Design review of the part built by this model. Coordinates are the model's own, in mm. Face numbers are marked on the shaded views. Round coordinates to 2 decimals unless told otherwise and drop trailing zeros. Order: outer loops, then holes, each group sorted by start corner. A loop starts at its lowest first (then second) coordinate and runs counter-clockwise, first axis right, second up. Notation, with made-up numbers: (-38, -9.5) - (-21, -9.5) arc R37 ccw to (-21, 29.5) - close; hole circle Ø1 at (-22.5, 45). An arc over 180 degrees is marked (long way). Write item = value, one per line.
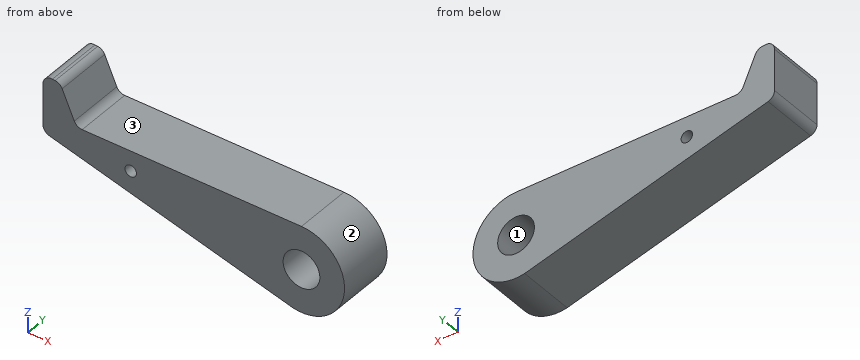
from build123d import *

# Parameters (mm, degrees)
SKETCH1_R           = 3.2
SKETCH1_R_2         = 1
BOSS_EXTRUDE1_DEPTH = 10
FILLET1_R           = 1.5


with BuildPart() as part:
    # Sketch1 → Boss-Extrude1 (new body)
    with BuildSketch(Plane(origin=(0, 0, 0), x_dir=(1, 0, 0), z_dir=(0, 1, 0))):
        with BuildLine():
            Line((0, 45), (43.494782903, 56.541397673))
            ThreePointArc((43.494782903, 56.541397673), (52.461753069, 49.950461527), (45, 41.69399531))
            Line((45, 41.69399531), (5.847258058, 41.69399531))
            Line((5.847258058, 41.69399531), (2.984330404, 35.306222204))
            Line((2.984330404, 35.306222204), (0, 35))
            Line((0, 35), (0, 45))
        make_face()
        with Locations(Location((45, 49.19399531, 0), (0, 0, 270))):
            Circle(SKETCH1_R, mode=Mode.SUBTRACT)
        with Locations(Location((15.270504009, 45.174409747, 0), (0, 0, 270))):
            Circle(SKETCH1_R_2, mode=Mode.SUBTRACT)
    extrude(amount=BOSS_EXTRUDE1_DEPTH)

    # Fillet1
    fillet1_edges = [part.edges().sort_by_distance(p)[0] for p in [
        (5.847258058, 5, -41.69399531),
        (2.984330404, 5, -35.306222204),
        (0, 5, -35),
        (0, 5, -45),
    ]]
    fillet(fillet1_edges, radius=FILLET1_R)


solid = part.part
Item 1: Take a section at A-A, the plane y = 1.25. State the section outline as (x, z) points, and give its area (3 significant figures).
Data:
outline = (0, -43.85) arc R1.5 ccw to (1.12, -45.3) - (43.49, -56.54) arc R7.5 ccw (long way) to (45, -41.69) - (6.82, -41.69) arc R1.5 cw to (5.45, -40.81) - (3.34, -36.1) arc R1.5 ccw to (2.12, -35.22) - (1.65, -35.17) arc R1.5 ccw to (0, -36.66) - close; hole circle Ø2 at (15.27, -45.17); hole circle Ø6.4 at (45, -49.19)
area = 498 mm2
Item 2: Take a section at C-C, the plane x = 39. State the section outline as (y, z) points, and give its area (3 significant figures).
Data:
outline = (0, -55.35) - (10, -55.35) - (10, -41.69) - (0, -41.69) - close
area = 137 mm2
Item 3: Insertion check: P1, Ø1.5, axis at x = 40, y = 5, coming from the -Z side; P2, Ø3, axis at y = 8, z = -46.5, coming from the +X side; P3, Ø5, axis at x = 18.5, y = 7, coming from the +Z side; P4, Ø7.5, axis at x = 45, z = -49.19, coming from the -Y side. Each pin has a flat end and moves straight along its axis. Give the tip position at first contact, or say it passes through.
Data:
P1 = -55.81
P2 = 52.4
P3 = -41.69
P4 = 0
Item 4: For line 1 along Z through (x, y) = (46, 5); line 2 along X through (y, z) = (7.25, -44.75); line 3 along Z through (x, y) = (26, 9), list the stretches that pass through material, from the lowest coordinate up. Write a range as [from, to].
Data:
line_1 = [-56.63, -52.23], [-46.15, -41.76]
line_2 = [0.3, 14.37], [16.18, 51.04]
line_3 = [-51.9, -41.69]
Item 5: Take a section at B-B, the plane z = -48.5. State the section outline as (x, y) points, and give its area (3 significant figures).
Data:
outline = (13.19, 0) - (41.88, 0) - (41.88, 10) - (13.19, 10) - close; (48.12, 0) - (52.47, 0) - (52.47, 10) - (48.12, 10) - close
area = 330 mm2
Item 6: Take a section at D-D, the plane z = -53.75. State the section outline as (x, y) points.
Data:
outline = (32.98, 0) - (50.96, 0) - (50.96, 10) - (32.98, 10) - close
Item 7: The part is to be moulded in two halves that separate along Z. For the marked faces 1, 2 and 3, say which applies: +Z half, -Z half, draft (parallel to the pull), parting line (faces both ways), or undercut.
Data:
face_1 = undercut
face_2 = parting line
face_3 = +Z half
